The listing builds one solid part. Answer for the finished solid, in the listing's coordinates (mm). A direction names the side the tool comes from. Round coordinates to 2 decimals unless told otherwise and drop trailing zeros. Order: outer loops, then holes, each group sorted by start corner. A loop starts at its lowest first (then second) coordinate and runs counter-clockwise, first axis right, second up. Notation, with made-up numbers: M -10,26 L 43,26 A17 ccw 43,52 Z; hole C -6,16.25 d7. An arc over 180 degrees is marked long. Write item = value, one per line. Start each with the question number.
(1) For a pull along Z with two mould halves and no side action, classify faces 1 (the face through (-87.253, 9.875, 86.66)), 2 (the face through (-88.594, 4.056, -87.972)), 3 (the face through (-18.86, 57.89, 20.76)), 4 (the face through (5, 30, -46)) as released by +Z, released by -Z, zero draft, split by the parting line, or undercut.
(2) Each of these flat-tipped pins is pushed along its axis until it touches: pin 1 (6 mm diameter, centred on x = -0.5, z = 45, fed in from +Y); pin 2 (4 mm diameter, centred on x = 28.5, z = -23.5, fed in from +Y); pin 3 (10 mm diameter, centred on y = 71, z = -4, fed in from -X). Where does it stop, or does it pass through?
(3) A cutting plane is placed at C-C, the plane y = 53. Determine the outline of the cut face in (x, z), and give its area (3 significant figures).
(4) A cutting plane is placed at B-B, the plane z = -62.5. Count the separate pieces of the cut face and the enclosed holes in it, and give its area (3 significant figures).
(5) Straight lines are drawn through the part: probe 1 along X at (y, z) = (3, -62); probe 2 along Y at (x, z) = (-40, 83.5); probe 3 along Z at (x, y) = (44.5, 33). For each, find the intervals that lie inside material, in ascending order. Write a range as from..to.
(6) Which of the six approach directions +Z, -Z, +X, -X, +Y, -Y give full straight-line access (tool end or side, diameter ignored) to faces 5 (the face through (-46, 30, -5)), 6 (the face through (46, 30, -5)), 7 (the face through (5, 30, 46))?
(7) A cutting plane is placed at A-A, the plane y = 32. Determine the outline of the cut face in (x, z), and give its area (3 significant figures).
from build123d import *

# Parameters (mm, degrees)
SKETCH2_W                       = 200
SKETCH2_H                       = 200
BOSS_EXTRUDE1_DEPTH             = 10
SKETCH3_R                       = 32.5
SKETCH3_R_2                     = 25
BOSS_EXTRUDE2_DEPTH             = 75
M10_CLEARANCE_HOLE1_D           = 11
M10_CLEARANCE_HOLE1_CSINK_D     = 13.5
M10_CLEARANCE_HOLE1_CSINK_ANGLE = 90
CIRPATTERN1_COUNT               = 2
CIRPATTERN1_ANGLE               = 90
RIB5_REACH                      = 167
SKETCH13_WALL_W                 = 401.282032406
SKETCH13_WALL_H                 = 10
CIRPATTERN2_COUNT               = 4
FILLET1_R                       = 25
FILLET2_R                       = 40
CHAMFER1_SIZE                   = 2


# Read off the part's stored shape, not the designer's step: M6x1.0 Tapped Hole1
with BuildPart() as part:
    # Sketch2 → Boss-Extrude1 (new body)
    with BuildSketch(Plane(origin=(0, 0, 0), x_dir=(1, 0, 0), z_dir=(0, 1, 0))):
        Rectangle(SKETCH2_W, SKETCH2_H)
    extrude(amount=BOSS_EXTRUDE1_DEPTH)

    # Sketch3 → Boss-Extrude2 (add)
    with BuildSketch(Plane(origin=(0, 10, 0), x_dir=(1, 0, 0), z_dir=(0, 1, 0))):
        with Locations(Location((0, 0, 0), (0, 0, 90))):
            Circle(SKETCH3_R)
        with Locations(Location((0, 0, 0), (0, 0, 270))):
            Circle(SKETCH3_R_2, mode=Mode.SUBTRACT)
    extrude(amount=BOSS_EXTRUDE2_DEPTH)

    # M10 Clearance Hole1 (through all)
    with Locations(Plane(origin=(0, 10, 0), x_dir=(1, 0, 0), z_dir=(0, 1, 0))):
        with Locations((-62.5, -62.5), (62.5, 62.5), (-62.5, 62.5), (62.5, -62.5)):
            CounterSinkHole(M10_CLEARANCE_HOLE1_D / 2, M10_CLEARANCE_HOLE1_CSINK_D / 2, counter_sink_angle=M10_CLEARANCE_HOLE1_CSINK_ANGLE)

    # M6x1.0 Tapped Hole1 outline → M6x1.0 Tapped Hole1 (revolve, cut)
    with BuildSketch(Plane(origin=(0, 60, 0), x_dir=(0.707106781186546, 0, 0.707106781186549), z_dir=(0, 1, 0))):
        Polygon((0, -32.500112934), (3.750112934, -32.500112934), (2.5, -31.25), (2.5, -24.874618187), (0, -24.874618187), align=None)
    m6x1_0_tapped_hole1 = revolve(axis=Axis((0, 60, 0), (0.707106781186549, 0, -0.707106781186546)), mode=Mode.SUBTRACT)

    # CirPattern1: M6x1.0 Tapped Hole1 ×2 about axis
    cirpattern1_axis = Axis((0, 85, 0), (0, -1, 0))
    for i in range(1, CIRPATTERN1_COUNT):
        add(m6x1_0_tapped_hole1.rotate(cirpattern1_axis, i * CIRPATTERN1_ANGLE / (CIRPATTERN1_COUNT - 1)), mode=Mode.SUBTRACT)

    # Sketch13 wall → Rib5 (add, up to next)
    with BuildSketch(Plane(origin=(-49.820508076, 40, 0), x_dir=(-0.499999999996, -0.866025403787, 0), z_dir=(0.866025403787, -0.499999999996, 0)), mode=Mode.PRIVATE) as rib5_sk1:
        Rectangle(SKETCH13_WALL_W, SKETCH13_WALL_H)
    rib5_tool1 = extrude(rib5_sk1.sketch, amount=RIB5_REACH, mode=Mode.PRIVATE) - part.part
    rib5 = rib5_tool1.solids().sort_by_distance((-49.820508076, 40, 0))[0]
    add(rib5)

    # CirPattern2: Rib5 ×4 about axis
    cirpattern2_axis = Axis((0, 0, 0), (0, 1, 0))
    for i in range(1, CIRPATTERN2_COUNT):
        add(rib5.rotate(cirpattern2_axis, i * 360 / CIRPATTERN2_COUNT))

    # Fillet1
    fillet1_edges = [part.edges().sort_by_distance(p)[0] for p in [
        (-22.980970389, 10, -22.980970389),
        (22.980970389, 10, -22.980970389),
        (22.980970389, 10, 22.980970389),
        (-22.980970389, 10, 22.980970389),
    ]]
    fillet(fillet1_edges, radius=FILLET1_R)

    # Fillet2
    fillet2_edges = [part.edges().sort_by_distance(p)[0] for p in [
        (100, 5, 100),
        (-100, 5, 100),
        (-100, 5, -100),
        (100, 5, -100),
    ]]
    fillet(fillet2_edges, radius=FILLET2_R)

    # Chamfer1
    chamfer1_edges = [part.edges().sort_by_distance(p)[0] for p in [
        (0, 10, 100),
        (-100, 10, 0),
        (0, 10, -100),
        (100, 10, 0),
        (88.284271247, 10, 88.284271247),
        (88.284271247, 10, -88.284271247),
        (-88.284271247, 10, -88.284271247),
        (-88.284271247, 10, 88.284271247),
    ]]
    chamfer(chamfer1_edges, length=CHAMFER1_SIZE)


solid = part.part
Reported:
q1.face_1 = released by +Z
q1.face_2 = released by -Z
q1.face_3 = undercut
q1.face_4 = zero draft
q2.pin_1 = 53.55
q2.pin_2 = 24.23
q2.pin_3 = -34.81
q3.outline = M -42.31,-5 L -32.11,-5 A32.5 ccw -5,-32.11 L -5,-42.31 L 5,-42.31 L 5,-32.11 A32.5 ccw 32.11,-5 L 42.31,-5 L 42.31,5 L 32.11,5 A32.5 ccw 5,32.11 L 5,42.31 L -5,42.31 L -5,32.11 A32.5 ccw -32.11,5 L -42.31,5 Z; hole C 0,0 d50
q3.area = 1,750 mm²
q4.separate_pieces = 3
q4.enclosed_holes = 0
q4.area = 1,850 mm²
q5.probe_1 = -99.95..-67.98, -57.02..57.02, 67.98..99.95
q5.probe_2 = 0..10
q5.probe_3 = -5..5
q6.face_5 = -Z, -X, +Y
q6.face_6 = -Z, +X, +Y
q6.face_7 = +Z, +X, +Y
q7.outline = M -54.44,-5 L -32.3,-5 A32.68 ccw -5,-32.3 L -5,-54.44 L 5,-54.44 L 5,-32.3 A32.68 ccw 32.3,-5 L 54.44,-5 L 54.44,5 L 32.3,5 A32.68 ccw 5,32.3 L 5,54.44 L -5,54.44 L -5,32.3 A32.68 ccw -32.3,5 L -54.44,5 Z; hole C 0,0 d50
q7.area = 2,270 mm²
